Can you work these out from the model? Positions are in its coordinate system, mm. A direction names the side the tool comes from. Give positions to 0.01 mm unless a question says otherwise; leave off trailing zeros. Write each loop counter-clockwise with the first axis right and the second up, starting at its lowest first coordinate (ties: lowest second). Pieces come first, ordered by that corner, then holes. Notation, with made-up numbers: M 22.5,-17 L 47.5,-17 A24 cw 47.5,3 Z; hole C 12.25,-37.75 d6. An arc over 180 degrees is marked long. Write each question's results on one line, items separated by ' | '.
from build123d import *

# Parameters (mm, degrees)
F0_R     = 63.5
F1_DEPTH = 127
F1_TAPER = -20
F2_R     = 19.4741575124
F3_SIZE  = 63.5
F4_T     = -12.7


# Not quite as in the source:
# - a shell that OpenCascade refuses in one call is made with other operations: the cavity is built on its own and cut out


with BuildPart() as f1:
    # F0 (on Front) → F1 (new body, symmetric)
    with BuildSketch(Plane.XZ):
        Circle(F0_R)
    extrude(amount=F1_DEPTH, both=True, taper=F1_TAPER)

    # F2
    f2_edges = [f1.edges().sort_by_distance(p)[0] for p in [
        (-109.72422, -127, 0),
    ]]
    fillet(f2_edges, radius=F2_R)

    # F3
    f3_edges = [f1.edges().sort_by_distance(p)[0] for p in [
        (-109.72422, 127, 0),
    ]]
    chamfer(f3_edges, length=F3_SIZE)

    # F4: a shell. OpenCascade refuses it in one call, so the cavity is built on its own and cut out:
    # the body offset inwards by the wall thickness, plus a prism from it out through each open face.
    f4_core = offset(f1.part, amount=F4_T, kind=Kind.INTERSECTION, mode=Mode.PRIVATE)
    f4_exits = [f4_core.faces().sort_by_distance(p)[0] for p in [
        (0, -114.3, 0),
    ]]
    add(f4_core, mode=Mode.SUBTRACT)
    extrude(f4_exits, amount=-F4_T, mode=Mode.SUBTRACT)


solid = f1.part
Item 1: I'm going to push flat-ended pins straight in: pin 1 (8 mm diameter, centred on y = -99, z = 73.5, fed in from +X); pin 2 (10 mm diameter, centred on y = -40.5, z = -67.5, fed in from -X); pin 3 (3 mm diameter, centred on y = 84, z = 2.5, fed in from -X). Where does each tip first touch, or does it pass through?
Geometry says:
pin 1: stops at x = 71.75 | pin 2: stops at x = -47.72 | pin 3: stops at x = -77.34
Item 2: Thinking about a two-plate mould opening in Z: for faces 4 (the face through (-17.757, -120.561, 79.964)), 5 (the face through (-14.688, 11.693, -66.145)), 6 (the face through (-1, 127, 1)), which applies, +Z half, -Z half, draft (parallel to the pull), parting line (faces both ways), or undercut?
Geometry says:
face 4: undercut | face 5: parting line | face 6: draft
Item 3: If I drill on line 1 (X direction, y = -16.5, z = -17.5); line 2 (Z direction, x = 0, y = -122); line 3 (X direction, y = -118.5, z = 0), over which ranges is the centre line in solid material (lowest first)? Write a range as from..to.
Geometry says:
line 1: x = -67.27..-53.19, 53.19..67.27 | line 2: z = -94.94..-81.91, 81.91..94.94 | line 3: x = -98..-81.91, 81.91..98
Item 4: I want a section at C-C, the plane y = 28. Please give me the cut outline in (x, z), and give its area (3 significant figures).
Geometry says:
outline: C 0,0 d147.38; hole C 0,0 d120.35 | area: 5,680 mm2
Item 5: I want a section at A-A, the plane z = -65. Give the number of separate pieces and of enclosed holes in the cut face, and give its area (3 significant figures).
Geometry says:
separate pieces: 2 | enclosed holes: 1 | area: 11,600 mm2
Item 6: I want a section at B-B, the plane x = 0. Please give me the cut outline in (y, z), and give its area (3 significant figures).
Geometry says:
outline: M -127,-81.91 A19.47 ccw -100.87,-100.21 L 0,-63.5 L 67.33,-88.01 L 127,-46.22 L 127,46.22 L 67.33,88.01 L 0,63.5 L -100.87,100.21 A19.47 ccw -127,81.91 L -114.3,81.91 A6.77 cw -105.21,88.28 L 0,49.98 L 65.46,73.81 L 114.3,39.61 L 114.3,-39.61 L 65.46,-73.81 L 0,-49.98 L -105.21,-88.28 A6.77 cw -114.3,-81.91 Z | area: 7,990 mm2
Item 7: For faces 1 (the face through (-1, 114.3, 1)), 2 (the face through (-5.37, 111.93, 40.92)), 3 (the face through (46.025, 124.103, 14.494)), which set-ups out of +Z, -Z, +X, -X, +Y, -Y let a thin tool reach every point of the face, with its end or its side?
Geometry says:
face 1: -Y | face 2: none | face 3: +Y
Item 8: I want a section at D-D, the plane y = -75. Please give me the cut outline in (x, z), and give its area (3 significant figures).
Geometry says:
outline: C 0,0 d181.6; hole C 0,0 d154.57 | area: 7,140 mm2
